Check sheet for the modelled part. Datum: model origin and axes. Units: mm. A direction names the side the tool comes from. Give positions to 0.01 mm unless a question says otherwise; leave off trailing zeros. Write each loop counter-clockwise with the first axis right and the second up, starting at its lowest first coordinate (ties: lowest second). Pieces come first, ordered by that corner, then holes. Notation, with made-up numbers: (-5.75, 36) -> (9.25, 36) arc R9 ccw to (9.25, 51) -> close; hole circle Ø8 at (-28.75, -10). An arc over 180 degrees is marked (long way). Return JSON: item names as keys, results as strings.
from build123d import *

# Parameters (mm, degrees)
F0_R      = 13.503105
F0_W      = 14.827031
F0_H      = 19.582872
F1_DEPTH  = 25.4
F1_FACE_R = 13.503105
F2_DEPTH  = 25.4
F3_W      = 30.36912
F3_H      = 79.002336
F4_DEPTH  = 25.4


with BuildPart() as f1:
    # F0 (on Front) → F1 (new body)
    with BuildSketch(Plane.XZ):
        Polygon((48.117902, -38.046706), (48.117902, 62.105667), (-17.778635, 62.105667), (-17.778635, -38.046706), (25.177971, -38.046706), (40.005002, -38.046706), align=None)
        with Locations((14.270158, 38.039379)):
            Circle(F0_R, mode=Mode.SUBTRACT)
        with Locations((32.591487, -47.838142)):
            Rectangle(F0_W, F0_H)
    extrude(amount=F1_DEPTH)

    # F1_face (on face) → F2 (join)
    with BuildSketch(Plane(origin=(16.051946, -25.4, 6.919351), x_dir=(1, 0, 0), z_dir=(0, -1, 0))):
        Polygon((32.065956, -44.966058), (32.065956, 55.186316), (-33.830581, 55.186316), (-33.830581, -44.966058), (9.126024, -44.966058), (9.126024, -64.548929), (23.953056, -64.548929), (23.953056, -44.966058), align=None)
        with Locations((-1.781788, 31.120028)):
            Circle(F1_FACE_R, mode=Mode.SUBTRACT)
    extrude(amount=F2_DEPTH)

    # F3 (on Right) → F4 (join)
    with BuildSketch(Plane.YZ):
        with Locations((15.18456, -39.501168)):
            Rectangle(F3_W, F3_H)
    extrude(amount=F4_DEPTH)


solid = f1.part
(1) Release check for a two-part mould opening along Y. For faces 1 (the flat face through (15, -50.8, 3)), 2 (the flat face through (16, -25, 62.106)) record: pulls with the +Y half, pulls with the -Y half, needs draft (parallel to the pull), parting line crosses it, or undercut.
Reply:
{"face 1": "pulls with the -Y half", "face 2": "needs draft"}
(2) Thickness scan on L1, parallel to Y at x = 2, z = -63; L2, parallel to Z at x = 14.5, y = 14.5; L3, parallel to X at y = -26, z = 31. Record the ranges inside material, lowest first.
Reply:
{"L1": "0 to 30.37", "L2": "-79 to 0", "L3": "-17.78 to 2.75, 25.79 to 48.12"}
(3) Set-up check for faces 3 (the flat face through (0, 15, -39)), 4 (the flat face through (25.4, 15, -39)), 5 (the flat face through (25.178, -38, -48)), 6 (the flat face through (44, -13, -38.047)): record each of +Z, -Z, +X, -X, +Y, -Y from which the full face is reachable in a straight line by a thin tool's end or side.
Reply:
{"face 3": "+Z, -Z, -X, +Y", "face 4": "+Z, -Z, +X, +Y", "face 5": "-Z, -X, -Y", "face 6": "-Z, +X, +Y, -Y"}
(4) Depth check by flat-ended pin: pin 1 Ø1.5 at (x, y) = (22, -5.5) entering from -Z; pin 2 Ø6 at (y, z) = (-9, -49.5) entering from -X; pin 3 Ø20.5 at (x, y) = (17, 13) entering from +Z. Enter the tip coordinate at first touch or a pass-through.
Reply:
{"pin 1": "z = -38.05", "pin 2": "x = 25.18", "pin 3": "z = 0"}
(5) Cross-section at A-A on z = -4.5. Enter the section's corners in (x, y), then the cut area to 3 significant figures.
Reply:
{"outline": "(-17.78, -50.8) -> (48.12, -50.8) -> (48.12, 0) -> (25.4, 0) -> (25.4, 30.37) -> (0, 30.37) -> (0, 0) -> (-17.78, 0) -> close", "area": "4,120 mm^2"}
(6) Cross-section at D-D on y = 20. Enter the section's corners in (x, z), then the cut area to 3 significant figures.
Reply:
{"outline": "(0, -79) -> (25.4, -79) -> (25.4, 0) -> (0, 0) -> close", "area": "2,010 mm^2"}
